Part model, mm, in its own coordinate system. A direction names the side the tool comes from. Round coordinates to 2 decimals unless told otherwise and drop trailing zeros. Loops run counter-clockwise (first coordinate to the right, second up) from the corner with the lowest first, then second, coordinate; pieces in that order, holes last. Notation, with made-up numbers: (-31.5, 41) - (-25.5, 41) arc R8 cw to (-25.5, 54) - close; hole circle Ø4 at (32.25, -1.5). An arc over 180 degrees is marked (long way). Write each question's results on one line, items separated by ' | '. Start each with the question number.
(1) Cut at A-A, the plane y = -92. List the corners of the cut face in (x, z).
(2) Cut at B-B, the plane x = -6.5. List the corners of the cut face in (y, z).
(3) Cut at C-C, the plane z = 20.5. List the corners of the cut face in (x, y).
(4) Drill centre lines: L1, parallel to Y at x = 4, z = 25; L2, parallel to X at y = -49, z = 23; L3, parallel to Z at x = 17, y = -71. Where is each one in solid material? Low to high.
(5) Tool access for faces 1 (the face through (0.4, 0, -0.4)), 2 (the face through (0, -49, 15)): list every direction of +Z, -Z, +X, -X, +Y, -Y with a clear straight run to the whole face (end or side of a thin tool).
(6) Flat gauge pins, fed straight in: P1, Ø3, axis at y = -22, z = 21.5, coming from the +X side; P2, Ø4, axis at y = -15.5, z = 18, coming from the -X side; P3, Ø4, axis at y = -23, z = 16, coming from the +X side. Where does each tip first touch, or does it go through?
from build123d import *

# Parameters (mm, degrees)
F1_DEPTH = 100
F2_R     = 5
F3_R     = 5


with BuildPart() as f1:
    # F0 (on Front) → F1 (new body)
    with BuildSketch(Plane.XZ):
        Polygon((0, 29.845397), (0, 0), (-29.831411, 0), (-29.831411, -20), (20.16835, -20.15432), (20, 29.845397), align=None)
    extrude(amount=F1_DEPTH)

    # F2
    f2_edges = [f1.edges().sort_by_distance(p)[0] for p in [
        (10, -100, 29.845397),
    ]]
    fillet(f2_edges, radius=F2_R)

    # F3
    f3_edges = [f1.edges().sort_by_distance(p)[0] for p in [
        (-29.831411, -100, -10),
    ]]
    fillet(f3_edges, radius=F3_R)


solid = f1.part
A:
1) outline: (-29.83, -20) - (20.17, -20.15) - (20, 29.85) - (0, 29.85) - (0, 0) - (-29.83, 0) - close
2) outline: (-100, -20.07) - (0, -20.07) - (0, 0) - (-100, 0) - close
3) outline: (0, -100) - (20.03, -100) - (20.03, 0) - (0, 0) - close
4) L1: -100 to 0 | L2: 0 to 20.02 | L3: -20.14 to 29.85
5) face 1: +Z, -Z, +X, -X, +Y | face 2: +Z, -X, +Y, -Y
6) P1: x = 20.03 | P2: x = 0 | P3: x = 20.05
